from build123d import *

# Parameters (mm, degrees)
IZIM1_W                     = 5
IZIM1_H                     = 2
IZIM3_W                     = 5
IZIM3_H                     = 2
IZIM3_W_2                   = 7
IZIM3_H_2                   = 4
Y_KSEKLIK_EKSTR_ZYON1_DEPTH = 2


with BuildPart() as part:
    # Süpür1: sweep along a path in Çizim2
    with BuildLine(Plane(origin=(0, 0, 0), x_dir=(0, 0, -1), z_dir=(1, 0, 0))) as s_p_r1_path:
        ThreePointArc((0, 0), (2.242898882, -14.32797835), (12.06275188, -25))
    # Çizim1 → Süpür1 (sweep)
    with BuildSketch(Plane(origin=(0, 0, 0), x_dir=(1, 0, 0), z_dir=(0, 1, 0))):
        with Locations((2.5, 1)):
            Rectangle(IZIM1_W, IZIM1_H)
    sweep(path=s_p_r1_path.line)

    # Çizim3 → Yükseklik-Ekstrüzyon1 (add)
    with BuildSketch(Plane(origin=(0, 0, 0), x_dir=(1, 0, 0), z_dir=(0, 1, 0))):
        with Locations((2.5, 1)):
            Rectangle(IZIM3_W, IZIM3_H)
        with Locations((2.5, 1)):
            Rectangle(IZIM3_W_2, IZIM3_H_2)
        with Locations((2.5, 1)):
            Rectangle(IZIM3_W, IZIM3_H, mode=Mode.SUBTRACT)
        with Locations((2.5, 1)):
            Rectangle(IZIM3_W, IZIM3_H)
    extrude(amount=Y_KSEKLIK_EKSTR_ZYON1_DEPTH)


solid = part.part
Work out the finished part from the listing and answer in its coordinate system (mm). A direction names the side the tool comes from. Give positions to 0.01 mm unless a question says otherwise; leave off trailing zeros. Order: outer loops, then holes, each group sorted by start corner. A loop starts at its lowest first (then second) coordinate and runs counter-clockwise, first axis right, second up. Notation, with made-up numbers: M -13.5,22 L 11.5,22 A22 cw 11.5,38 Z; hole C -11.75,-28.75 d10. An arc over 180 degrees is marked long. Return JSON: item names as keys, results as strings.
Q1. Find section D-D, the plane z = -4.75. Write down the section's boundary in (x, y).
Answer below:
{"outline": "M 0,-18.45 L 5,-18.45 L 5,-14.85 L 0,-14.85 Z"}
Q2. The mould has two halves that part along Y. Classify faces 4 (the face through (2.46, -13.05, -3.83)), 5 (the face through (2, 1, -3)), 6 (the face through (2.5, 0, -2.4)), 7 (the face through (2.46, -24.09, -12.44)): pulls with the +Y half, pulls with the -Y half, needs draft (parallel to the pull), parting line crosses it, or undercut.
Answer below:
{"face 4": "undercut", "face 5": "needs draft", "face 6": "undercut", "face 7": "pulls with the -Y half"}
Q3. Each of these flat-tipped pins is pushed along its axis until it touches: pin 1 (1 mm diameter, centred on y = -6.5, z = -3.5, fed in from -X); pin 2 (1.5 mm diameter, centred on x = 0.5, y = -8.5, fed in from -Z); pin 3 (0.6 mm diameter, centred on x = 1, y = 0.5, fed in from -Z); pin 4 (1.2 mm diameter, centred on x = 3.5, z = -2, fed in from -Y). Where does it stop, or does it pass through?
Answer below:
{"pin 1": "passes through", "pin 2": "stops at z = -2.48", "pin 3": "stops at z = -3", "pin 4": "stops at y = -15.04"}
Q4. Which of the six approach directions +Z, -Z, +X, -X, +Y, -Y give full straight-line access (tool end or side, diameter ignored) to faces 1 (the face through (0, -14, -3)), 2 (the face through (-1, 1, -1)), 3 (the face through (5, -14, -4))?
Answer below:
{"face 1": "+Z, -Z, -X, -Y", "face 2": "+Z, -Z, -X, +Y, -Y", "face 3": "+Z, -Z, +X, -Y"}
Q5. Find the intervals of material crossed by line 1 along X through (y, z) = (-5.5, -1); line 2 along Z through (x, y) = (0.25, 0.5); line 3 along Y through (x, z) = (3.25, -9.5), in increasing order. Write a range as [from, to].
Answer below:
{"line 1": "x = [0, 5]", "line 2": "z = [-3, 1]", "line 3": "y = [-23.27, -20.7]"}
Q6. Find section A-A, the plane x = 4.75. Write down the section's boundary in (y, z), and give its area (3 significant figures).
Answer below:
{"outline": "M -25,-12.06 L -23.15,-12.83 A23.02 cw 0,-2 L 0,-3 L 2,-3 L 2,1 L 0,1 L 0,0 A25 ccw Z", "area": "63.9 mm^2"}
Q7. Find section C-C, the plane y = -2.5. Write down the section's boundary in (x, z), and give its area (3 significant figures).
Answer below:
{"outline": "M 0,-1.76 L 5,-1.76 L 5,0.22 L 0,0.22 Z", "area": "9.90 mm^2"}
Q8. Find section B-B, the plane z = -2.25. Write down the section's boundary in (x, y), and give its area (3 significant figures).
Answer below:
{"outline": "M -1,0 L 6,0 L 6,2 L -1,2 Z; M 0,-14.34 L 5,-14.34 L 5,-8.29 L 0,-8.29 Z", "area": "44.3 mm^2"}
